from build123d import *

# Parameters (mm, degrees)
SKETCH_1_W          = 35
SKETCH_1_H          = 32
SKETCH_1_R          = 3.5
EXTRUDE_1_DEPTH     = 2
SKETCH_2_R          = 1.55
CUT_EXTRUDE_1_DEPTH = 10


with BuildPart() as part:
    # 草图1 → 凸台-拉伸1 (new body)
    with BuildSketch(Plane(origin=(0, 0, 0), x_dir=(1, 0, 0), z_dir=(0, 1, 0))):
        Rectangle(SKETCH_1_W, SKETCH_1_H)
        with Locations(Location((0, 0, 0), (0, 0, 270))):
            Circle(SKETCH_1_R, mode=Mode.SUBTRACT)
        with BuildLine():
            Line((-1.55, 9.5), (-1.55, 8))
            ThreePointArc((-1.55, 8), (0, 6.45), (1.55, 8))
            Line((1.55, 8), (1.55, 9.5))
            ThreePointArc((1.55, 9.5), (0, 11.05), (-1.55, 9.5))
        make_face(mode=Mode.SUBTRACT)
        with BuildLine():
            Line((1.55, -9.5), (1.55, -8))
            ThreePointArc((1.55, -8), (0, -6.45), (-1.55, -8))
            Line((-1.55, -8), (-1.55, -9.5))
            ThreePointArc((-1.55, -9.5), (0, -11.05), (1.55, -9.5))
        make_face(mode=Mode.SUBTRACT)
        with BuildLine():
            Line((-9.5, -1.55), (-8, -1.55))
            ThreePointArc((-8, -1.55), (-6.45, 0), (-8, 1.55))
            Line((-8, 1.55), (-9.5, 1.55))
            ThreePointArc((-9.5, 1.55), (-11.05, 0), (-9.5, -1.55))
        make_face(mode=Mode.SUBTRACT)
        with BuildLine():
            Line((9.5, 1.55), (8, 1.55))
            ThreePointArc((8, 1.55), (6.45, 0), (8, -1.55))
            Line((8, -1.55), (9.5, -1.55))
            ThreePointArc((9.5, -1.55), (11.05, 0), (9.5, 1.55))
        make_face(mode=Mode.SUBTRACT)
    extrude(amount=EXTRUDE_1_DEPTH)

    # 草图2 → 切除-拉伸1 (cut)
    with BuildSketch(Plane(origin=(0, 2, 0), x_dir=(1, 0, 0), z_dir=(0, 1, 0))):
        with Locations(Location((-14.5, 13, 0), (0, 0, 270))):
            Circle(SKETCH_2_R)
        with Locations(Location((-14.5, -13, 0), (0, 0, 270))):
            Circle(SKETCH_2_R)
        with Locations(Location((14.5, -13, 0), (0, 0, 270))):
            Circle(SKETCH_2_R)
        with Locations(Location((14.5, 13, 0), (0, 0, 270))):
            Circle(SKETCH_2_R)
    extrude(amount=-CUT_EXTRUDE_1_DEPTH, mode=Mode.SUBTRACT)


solid = part.part
Geometry: final body of the model. Coordinates: model frame, mm. A direction names the side the tool comes from. Round coordinates to 2 decimals unless told otherwise and drop trailing zeros. Loops run counter-clockwise (first coordinate to the right, second up) from the corner with the lowest first, then second, coordinate; pieces in that order, holes last. Notation, with made-up numbers: (-9.5, -31.75) - (20.5, -31.75) arc R26 ccw to (20.5, -4.75) - close; hole circle Ø8 at (-15, 34.5). An arc over 180 degrees is marked (long way). Write each question's results on one line, items separated by ' | '. Start each with the question number.
1) Cut plane A-A on x = 14.5. Return loops of the section in (y, z), then the cut area to 3 significant figures.
2) Cut plane D-D on x = 0. Return loops of the section in (y, z), then the cut area to 3 significant figures.
3) Cut plane B-B on z = 0. Return loops of the section in (x, y).
4) Line query: probe 1 along X at (y, z) = (0.75, -13); probe 2 along X at (y, z) = (1.3, 0); probe 3 along Z at (x, y) = (15.5, 1.65). Output: solid intervals per line, ascending. Write a range as [from, to].
5) First-contact query: P1, Ø2.5, axis at x = 14.5, z = 13, coming from the -Y side; P2, Ø5, axis at x = -14.5, z = -13, coming from the -Y side. Flat tips, straight axial feed; report the tip coordinate or a pass-through.
6) Access query for faces 1 (the face through (17.5, 1, 0)), 2 (the face through (-1.55, 1, -9)). Directions: +Z, -Z, +X, -X, +Y, -Y. A direction counts if a zero-diameter tool reaches every point of the face in a straight line with its end or side. Return the directions, or none.
7) Cut plane C-C on y = 1.25. Count the separate pieces of the cut face and the enclosed holes in it, then the cut area to 3 significant figures.
Verdict:
1) outline: (0, -16) - (2, -16) - (2, -14.55) - (0, -14.55) - close; (0, -11.45) - (2, -11.45) - (2, 11.45) - (0, 11.45) - close; (0, 14.55) - (2, 14.55) - (2, 16) - (0, 16) - close | area: 51.6 mm2
2) outline: (0, -16) - (2, -16) - (2, -11.05) - (0, -11.05) - close; (0, -6.45) - (2, -6.45) - (2, -3.5) - (0, -3.5) - close; (0, 3.5) - (2, 3.5) - (2, 6.45) - (0, 6.45) - close; (0, 11.05) - (2, 11.05) - (2, 16) - (0, 16) - close | area: 31.6 mm2
3) outline: (-17.5, 0) - (-11.05, 0) - (-11.05, 2) - (-17.5, 2) - close; (-6.45, 0) - (-3.5, 0) - (-3.5, 2) - (-6.45, 2) - close; (3.5, 0) - (6.45, 0) - (6.45, 2) - (3.5, 2) - close; (11.05, 0) - (17.5, 0) - (17.5, 2) - (11.05, 2) - close
4) probe 1: x = [-17.5, -16.05], [-12.95, 12.95], [16.05, 17.5] | probe 2: x = [-17.5, -11.05], [-6.45, -3.5], [3.5, 6.45], [11.05, 17.5] | probe 3: z = [-16, -14.18], [-11.82, 11.82], [14.18, 16]
5) P1: passes through | P2: stops at y = 0
6) face 1: +Z, -Z, +X, +Y, -Y | face 2: +Y, -Y
7) separate pieces: 1 | enclosed holes: 9 | area: 1,000 mm2
